For this review, take the finished solid that the model builds, in its own axes (mm). Face numbers are marked on the shaded views. A direction names the side the tool comes from. Round coordinates to 2 decimals unless told otherwise and drop trailing zeros. Write each loop counter-clockwise with the first axis right and the second up, starting at its lowest first coordinate (ties: lowest second). Pieces come first, ordered by that corner, then holes.
from build123d import *

# Parameters (mm, degrees)
SKETCH1_R           = 1.5
BOSS_EXTRUDE1_DEPTH = 50
SKETCH3_R           = 1.5
CUT_EXTRUDE1_DEPTH  = 50


with BuildPart() as part:
    # Sketch1 → Boss-Extrude1 (new body)
    with BuildSketch(Plane.XY):
        with BuildLine():
            ThreePointArc((-438.463421682, 243.552927072), (-440.963421682, 246.052927072), (-443.463421682, 243.552927072))
            Line((-443.463421682, 243.552927072), (-443.463421682, 241.075715503))
            Line((-443.463421682, 241.075715503), (-443.553411549, 241.076505927))
            Line((-443.553411549, 241.076505927), (-529.959210098, 241.076505927))
            Line((-529.959210098, 241.076505927), (-529.959210098, 246.076505927))
            ThreePointArc((-529.959210098, 246.076505927), (-534.959210098, 251.076505927), (-539.959210098, 246.076505927))
            Line((-539.959210098, 246.076505927), (-544.959210098, 246.076505927))
            ThreePointArc((-544.959210098, 246.076505927), (-542.030277909, 239.005438115), (-534.959210098, 236.076505927))
            Line((-534.959210098, 236.076505927), (-441.589975913, 236.076505927))
            ThreePointArc((-441.589975913, 236.076505927), (-399.328149739, 226.70728463), (-364.985531601, 200.355266895))
            Line((-364.985531601, 200.355266895), (-359.959210098, 194.365130186))
            Line((-359.959210098, 194.365130186), (-271.489088985, 194.365130186))
            ThreePointArc((-271.489088985, 194.365130186), (-241.418509035, 198.993435111), (-214.13144535, 212.449925757))
            Line((-214.13144535, 212.449925757), (-156.452183895, 252.837379426))
            Line((-156.452183895, 252.837379426), (-157.855222331, 255.337379426))
            ThreePointArc((-157.855222331, 255.337379426), (-160.355222331, 257.837379426), (-162.855222331, 255.337379426))
            Line((-162.855222331, 255.337379426), (-165.169417873, 252.837379426))
            Line((-165.169417873, 252.837379426), (-216.999327532, 216.545685979))
            ThreePointArc((-216.999327532, 216.545685979), (-241.871536557, 204.099961997), (-269.282233437, 199.390766337))
            Line((-269.282233437, 199.390766337), (-269.282233437, 201.571985734))
            ThreePointArc((-269.282233437, 201.571985734), (-271.489088985, 203.778841282), (-273.695944534, 201.571985734))
            Line((-273.695944534, 201.571985734), (-273.695944534, 199.365130186))
            Line((-273.695944534, 199.365130186), (-353.961902661, 199.365130186))
            Line((-353.961902661, 199.365130186), (-353.961902661, 201.865130186))
            ThreePointArc((-353.961902661, 201.865130186), (-354.694135708, 203.632897139), (-356.461902661, 204.365130186))
            Line((-356.461902661, 204.365130186), (-361.829937067, 204.365130186))
            ThreePointArc((-361.829937067, 204.365130186), (-396.313657586, 230.813272806), (-438.553411549, 241.032588537))
            Line((-438.553411549, 241.032588537), (-438.463421682, 241.031798113))
            Line((-438.463421682, 241.031798113), (-438.463421682, 243.552927072))
        make_face()
        with Locations((-440.963421682, 243.552927072)):
            Circle(SKETCH1_R, mode=Mode.SUBTRACT)
        with Locations((-534.959210098, 246.076505927)):
            Circle(SKETCH1_R, mode=Mode.SUBTRACT)
        with Locations((-160.355222331, 255.337379426)):
            Circle(SKETCH1_R, mode=Mode.SUBTRACT)
        with Locations((-356.461902661, 201.865130186)):
            Circle(SKETCH1_R, mode=Mode.SUBTRACT)
    extrude(amount=BOSS_EXTRUDE1_DEPTH)

    # Sketch3 → Cut-Extrude1 (cut)
    with BuildSketch(Plane.XY.offset(50)):
        with Locations((-271.489088985, 201.571985734)):
            Circle(SKETCH3_R)
    extrude(amount=-CUT_EXTRUDE1_DEPTH, mode=Mode.SUBTRACT)


solid = part.part
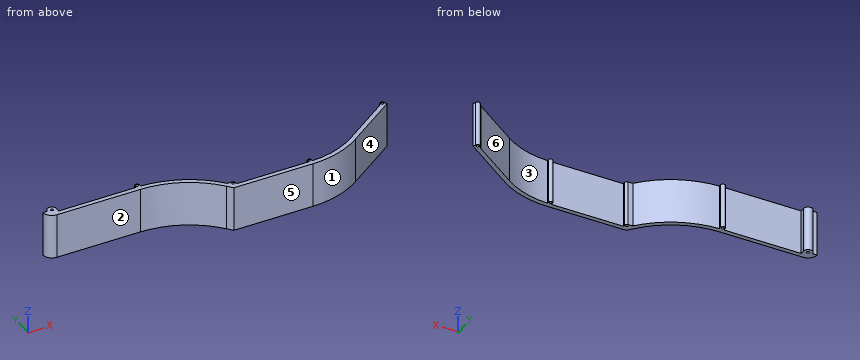
(1) For pin 1 Ø1 at (y, z) = (251, 10) entering from +X; pin 2 Ø5 at (y, z) = (209.5, 14.5) entering from +X; pin 3 Ø2.5 at (x, y) = (-271.49, 201.57) entering from +Z; pin 4 Ø0.7 at (y, z) = (241.5, 17.5) entering from -X, all flat-tipped, find the tip position at first contact; note any pin that passes through.
Geometry check:
pin 1: stops at x = -158.36
pin 2: stops at x = -214.78
pin 3: passes through
pin 4: stops at x = -544.02
(2) We need section B-B, the plane y = 223.5. Give the boundary of the cut face in (x, z), and give its area (3 significant figures).
Geometry check:
outline: (-393.04, 0) - (-383.43, 0) - (-383.43, 50) - (-393.04, 50) - close; (-207.07, 0) - (-198.35, 0) - (-198.35, 50) - (-207.07, 50) - close
area: 916 mm2
(3) Mouldability with a two-part tool opening along X and no side actions: class the marked faces 4, 5 and 6 as pulls with the +X half, pulls with the -X half, needs draft (parallel to the pull), parting line crosses it, or undercut.
Geometry check:
face 4: pulls with the +X half
face 5: needs draft
face 6: undercut
(4) For line 1 along Y through (x, z) = (-298.5, 28); line 2 along X through (y, z) = (220.5, 18); line 3 along X through (y, z) = (228.5, 19.5), list the stretches that pass through material, from the lowest coordinate up.
Geometry check:
line 1: y = 194.37 to 199.37
line 2: x = -387.99 to -379.16, -211.35 to -202.63
line 3: x = -403.41 to -391.76, -199.93 to -191.21
(5) For the marked faces 1, 2 and 3, list the 3-axis set-ups (+Z, -Z, +X, -X, +Y, -Y) from which the entire face can be reached by the end or side of a thin tool; tool diameter is ignored.
Geometry check:
face 1: +Z, -Z, +X, -Y
face 2: +Z, -Z, -X, -Y
face 3: +Z, -Z, +Y
(6) We need section D-D, the plane x = -378.5. Give the boundary of the cut face in (y, z).
Geometry check:
outline: (213.66, 0) - (220.01, 0) - (220.01, 50) - (213.66, 50) - close
(7) We need section C-C, the plane x = -500. Give the boundary of the cut face in (y, z), and give its area (3 significant figures).
Geometry check:
outline: (236.08, 0) - (241.08, 0) - (241.08, 50) - (236.08, 50) - close
area: 250 mm2
(8) We need section A-A, the plane z = 32. State how many separate pieces and enclosed holes the cut face has, and give its area (3 significant figures).
Geometry check:
separate pieces: 1
enclosed holes: 5
area: 2,220 mm2
